Read the model definition and answer for the solid it produces. Units are mm, in the model's axes. A direction names the side the tool comes from. Coordinates: 2 decimals unless noted, no trailing zeros. Write each loop counter-clockwise with the first axis right and the second up, starting at its lowest first coordinate (ties: lowest second). Pieces come first, ordered by that corner, then holes.
(1) Which of the six approach directions +Z, -Z, +X, -X, +Y, -Y give full straight-line access (tool end or side, diameter ignored) to faces 1 (the flat face through (-2, 0, 0.432)), 2 (the flat face through (-0.1, 10.414, 0.2))?
(2) Straight lines are drawn through the part: line 1 along X through (y, z) = (-3.5, 0.95); line 2 along X through (y, z) = (-1.75, 0.25); line 3 along Y through (x, z) = (1, 0.2). For each, find the intervals that lie inside material, in ascending order.
(3) The part is cut by section A-A, the plane x = -0.25. Determine the outline of the cut face in (y, z), and give its area (3 significant figures).
(4) The part is cut by section C-C, the plane x = 3.5. Determine the outline of the cut face in (y, z).
(5) Determine the mould class of faces 3 (the flat face through (-6.172, 0, 1)), 4 (the flat face through (7, 0, 1.448)), 5 (the flat face through (7.366, 0, 1)) for opening direction X: pulls with the +X half, pulls with the -X half, needs draft (parallel to the pull), parting line crosses it, or undercut.
(6) The part is cut by section B-B, the plane z = 0.8. Determine the outline of the cut face in (x, y).
(7) Given pin 1 (1.5 mm diameter, centred on x = 1, y = 4.5, fed in from +Z), flat-ended and moving along its own axis, determine where the tip first touches the part or whether it passes through.
```python
from build123d import *

# Parameters (mm, degrees)
F0_W     = 14.732
F0_H     = 20.828
F1_DEPTH = 0.4318
F2_W     = 0.127
F2_H     = 20.828
F3_DEPTH = 0.0762
F4_W     = 3.048
F4_H     = 9.144
F5_DEPTH = 25.4
F6_W     = 1.1938
F6_H     = 20.828
F7_DEPTH = 1.016


with BuildPart() as f1:
    # F0 (on Top) → F1 (new body)
    with BuildSketch(Plane.XY):
        Rectangle(F0_W, F0_H)
    extrude(amount=F1_DEPTH)

    # F2 (on face) → F3 (cut)
    with BuildSketch(Plane.XY.offset(0.4318)):
        with Locations((-5.3467, 0)):
            Rectangle(F2_W, F2_H)
        with Locations((-3.8227, 0)):
            Rectangle(F2_W, F2_H)
        with Locations((-2.2987, 0)):
            Rectangle(F2_W, F2_H)
        with Locations((-0.7747, 0)):
            Rectangle(F2_W, F2_H)
        with Locations((0.7493, 0)):
            Rectangle(F2_W, F2_H)
        with Locations((2.2733, 0)):
            Rectangle(F2_W, F2_H)
        with Locations((3.7973, 0)):
            Rectangle(F2_W, F2_H)
        with Locations((5.3213, 0)):
            Rectangle(F2_W, F2_H)
    extrude(amount=-F3_DEPTH, mode=Mode.SUBTRACT)

    # F4 (on face) → F5 (cut)
    with BuildSketch(Plane.XY.offset(0.4318)):
        Rectangle(F4_W, F4_H)
    extrude(amount=-F5_DEPTH, mode=Mode.SUBTRACT)

    # F6 (on face) → F7 (join)
    with BuildSketch(Plane.XY.offset(0.4318)):
        with Locations((-6.7691, 0)):
            Rectangle(F6_W, F6_H)
        with Locations((6.7691, 0)):
            Rectangle(F6_W, F6_H)
    extrude(amount=F7_DEPTH)


solid = f1.part
```
Computed:
1. face 1: +Z, +Y, -Y
1. face 2: +Z, -Z, +X, -X, +Y
2. line 1: x = -7.37 to -6.17, 6.17 to 7.37
2. line 2: x = -7.37 to -1.52, 1.52 to 7.37
2. line 3: y = -10.41 to -4.57, 4.57 to 10.41
3. outline: (-10.41, 0) - (-4.57, 0) - (-4.57, 0.43) - (-10.41, 0.43) - close; (4.57, 0) - (10.41, 0) - (10.41, 0.43) - (4.57, 0.43) - close
3. area: 5.05 mm2
4. outline: (-10.41, 0) - (10.41, 0) - (10.41, 0.43) - (-10.41, 0.43) - close
5. face 3: undercut
5. face 4: needs draft
5. face 5: pulls with the +X half
6. outline: (-7.37, -10.41) - (-6.17, -10.41) - (-6.17, 10.41) - (-7.37, 10.41) - close; (6.17, -10.41) - (7.37, -10.41) - (7.37, 10.41) - (6.17, 10.41) - close
7. pin 1: stops at z = 0.43
